Print and shaded views of the part. All mm, measured from the part's lowest x, y and z. Coordinates: 2 decimals unless noted, no trailing zeros. Order: outer loops, then holes, each group sorted by start corner. A loop starts at its lowest first (then second) coordinate and runs counter-clockwise, first axis right, second up. Notation, with made-up numbers: (32, 69.5) - (79, 69.5) arc R13 ccw to (79, 91.5) - close; hole circle Ø11 at (82, 31). An arc over 180 degrees is marked (long way). Write each question's results on one line, items separated by ' | '.
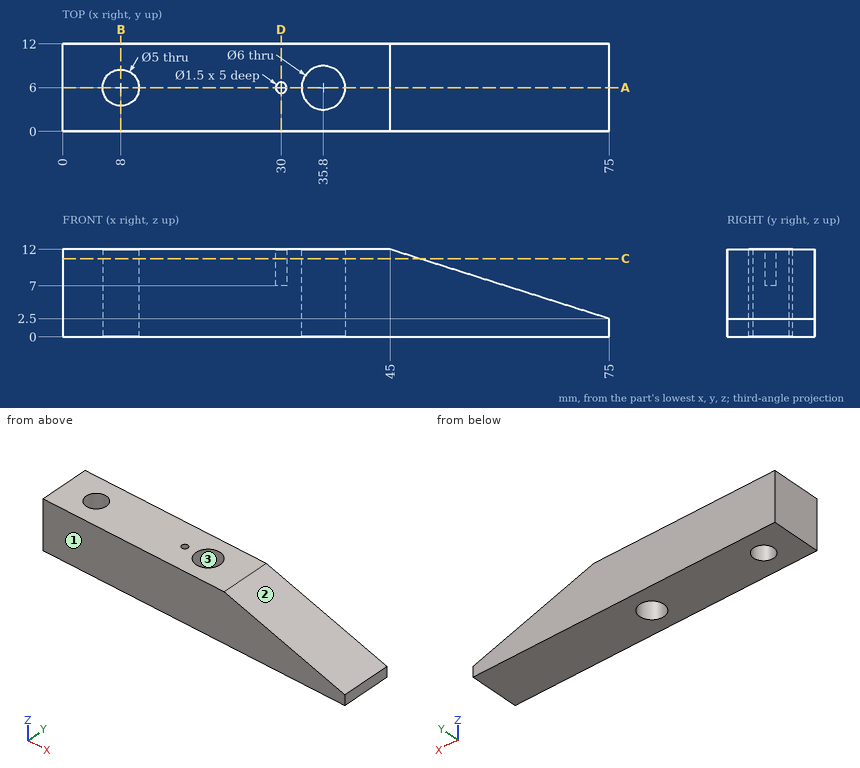
1. Drop flat-ended pins along their axis: pin 1 Ø4 at (x, y) = (8, 6) entering from +Z; pin 2 Ø1 at (y, z) = (5.5, 9) entering from -X; pin 3 Ø5 at (x, y) = (57.5, 5.5) entering from +Z; pin 4 Ø0.9 at (x, y) = (30, 6) entering from +Z. Give the stop position or say it passes through.
Solved:
pin 1: passes through | pin 2: stops at x = 0 | pin 3: stops at z = 8.83 | pin 4: stops at z = 7
2. Two-plate mould, pull along Y, no slides. Class the marked faces 1, 2 and 3: +Y half, -Y half, draft (parallel to the pull), parting line (faces both ways), or undercut.
Solved:
face 1: -Y half | face 2: draft | face 3: undercut
3. Probe line 1 (Y direction, x = 8, z = 3.25); line 2 (Y direction, x = 30, z = 8.15); line 3 (Z direction, x = 71, y = 9.5). List the from-to ranges inside material, lowest first.
Solved:
line 1: y = 0 to 3.5, 8.5 to 12 | line 2: y = 0 to 5.25, 6.75 to 12 | line 3: z = 0 to 3.77
4. Band-saw the part on B-B on x = 8. Give the cut face in (y, z).
Solved:
outline: (0, 0) - (3.5, 0) - (3.5, 12) - (0, 12) - close; (8.5, 0) - (12, 0) - (12, 12) - (8.5, 12) - close
5. Band-saw the part on D-D on x = 30. Give the cut face in (y, z).
Solved:
outline: (0, 0) - (12, 0) - (12, 12) - (6.75, 12) - (6.75, 7) - (5.25, 7) - (5.25, 12) - (0, 12) - close
6. Band-saw the part on C-C on z = 10.75. Give the cut face in (x, y), then the cut area to 3 significant figures.
Solved:
outline: (0, 0) - (48.95, 0) - (48.95, 12) - (0, 12) - close; hole circle Ø5 at (8, 6); hole circle Ø1.5 at (30, 6); hole circle Ø6 at (35.8, 6) | area: 538 mm2
7. Band-saw the part on A-A on y = 6. Give the cut face in (x, z), then the cut area to 3 significant figures.
Solved:
outline: (0, 0) - (5.5, 0) - (5.5, 12) - (0, 12) - close; (10.5, 0) - (32.8, 0) - (32.8, 12) - (30.75, 12) - (30.75, 7) - (29.25, 7) - (29.25, 12) - (10.5, 12) - close; (38.8, 0) - (75, 0) - (75, 2.5) - (45, 12) - (38.8, 12) - close | area: 618 mm2
